Verification items for the finished model (mm, model axes). Face numbers are marked on the shaded views. A direction names the side the tool comes from. Give positions to 0.01 mm unless a question says otherwise; leave off trailing zeros. Order: outer loops, then holes, each group sorted by start corner. A loop starts at its lowest first (then second) coordinate and runs counter-clockwise, first axis right, second up. Notation, with made-up numbers: (-37.5, 46) -> (8.5, 46) arc R20 cw to (8.5, 64) -> close; hole circle Ø11 at (74.25, 50). An arc over 180 degrees is marked (long way). One line per question, with ' | ' between items. Start each with the question number.
Q1. Go/stop test with flat-tipped pins: pin 1 (1 mm diameter, centred on x = 40, z = -6.5, fed in from -Y); pin 2 (5 mm diameter, centred on x = 60, y = 23.5, fed in from +Z); pin 3 (13.5 mm diameter, centred on x = 62.5, z = -3.5, fed in from +Y). Record where each tip stops, or that it passes through.
Q2. Material ranges on probe 1 along Y at (x, z) = (-16.5, 2); probe 2 along Y at (x, z) = (7, -6.5); probe 3 along X at (y, z) = (2.5, -8), recorded low to high. Write a range as [from, to].
Q3. Access from +Z, -Z, +X, -X, +Y, -Y to the whole of each face (thin tool, end or side, straight path). Record for the marked faces 5, 6 and 7.
Q4. Mould release check, pull along Y, two halves, no side actions. Record for the marked faces 1, 2, 3 and 4: released by +Y, released by -Y, zero draft, split by the parting line, or undercut.
Q5. Section check B-B on y = -35. Record the cut outline in (x, z), plus the area to 3 significant figures.
Q6. Section check A-A on x = 7. Record the cut outline in (y, z), plus the area to 3 significant figures.
from build123d import *

# Parameters (mm, degrees)
SKETCH001_W          = 113
SKETCH001_H          = 85
PAD001_DEPTH         = 25
POCKET_DEPTH         = 36.5
SKETCH003_W          = 67.1
SKETCH003_H          = 19.5
POCKET001_DEPTH      = 61.5
POCKET002_DEPTH      = 17.5
SKETCH005_W          = 4
SKETCH005_H          = 8
SKETCH005_W_2        = 10
SKETCH005_H_2        = 10
POCKET003_DEPTH      = 42.501
POCKET003_DEPTH_BACK = 42.501
SKETCH006_W          = 3.6
SKETCH006_H          = 6
POCKET004_DEPTH      = 17
SKETCH007_W          = 250
SKETCH007_H          = 80
POCKET005_DEPTH      = 112.501
SKETCH008_R          = 30
POCKET006_DEPTH      = 32
POCKET007_DEPTH      = 18.5
POCKET008_DEPTH      = 25
SKETCH012_W          = 37.5
SKETCH012_H          = 25
POCKET009_DEPTH      = 20
SKETCH026_W          = 5
SKETCH026_H          = 10
PAD008_DEPTH         = 5
POCKET014_DEPTH      = 63.501
POCKET015_DEPTH      = 15
SKETCH029_W          = 1.43005
SKETCH029_H          = 20
PAD009_DEPTH         = 20
POCKET016_DEPTH      = 9
CHAMFER_SIZE         = 3
POCKET017_DEPTH      = 15
SKETCH032_W          = 21
SKETCH032_H          = 11.5
POCKET018_DEPTH      = 41


with BuildPart() as part:
    # Sketch001 → Pad001 (new body, symmetric)
    with BuildSketch(Plane.XY):
        with Locations((26.5, 0)):
            Rectangle(SKETCH001_W, SKETCH001_H)
    extrude(amount=PAD001_DEPTH, both=True)

    # Sketch002 (on DatumPlane) → Pocket (cut)
    with BuildSketch(Plane.XZ.offset(70)):
        with BuildLine():
            ThreePointArc((0, -20), (10.954451, -16.733201), (18.330303, -8))
            Line((18.330303, -8), (55.5, -8))
            Line((55.5, -8), (55.5, 20))
            Line((55.5, 20), (-30, 20))
            Line((-30, 20), (-30, -20))
            Line((-30, -20), (0, -20))
        make_face()
    pocket = extrude(amount=-POCKET_DEPTH, mode=Mode.SUBTRACT)

    # Mirrored: Pocket across XZ
    add(pocket.mirror(Plane.XZ), mode=Mode.SUBTRACT)

    # Sketch003 (on DatumPlane) → Pocket001 (cut)
    with BuildSketch(Plane.XY.offset(50)):
        with Locations((21.95, -29.65)):
            Rectangle(SKETCH003_W, SKETCH003_H)
        with Locations((21.95, 29.65)):
            Rectangle(SKETCH003_W, SKETCH003_H)
    extrude(amount=-POCKET001_DEPTH, mode=Mode.SUBTRACT)

    # Sketch004 (on DatumPlane) → Pocket002 (cut, symmetric)
    with BuildSketch(Plane.XZ):
        Polygon((-21, 4.923702), (-9.5, -11.5), (77, -11.5), (77, 8.5), (74, 11.5), (74, 38.5), (-21, 38.5), (-21, 13.5), (-19, 13.5), (-19, 12.5), (-21, 10.5), align=None)
    extrude(amount=POCKET002_DEPTH, both=True, mode=Mode.SUBTRACT)

    # Sketch005 (on DatumPlane) → Pocket003 (cut, two sides)
    with BuildSketch(Plane.XZ) as pocket003_sk:
        with Locations((31, 0)):
            Rectangle(SKETCH005_W, SKETCH005_H)
        with Locations((50.5, 0)):
            Rectangle(SKETCH005_W_2, SKETCH005_H_2)
        with BuildLine():
            ThreePointArc((3.272614, 2.3), (-4, 0), (3.272614, -2.3))
            Line((11.25, -2.3), (3.272614, -2.3))
            ThreePointArc((11.25, -2.3), (13.55, 0), (11.25, 2.3))
            Line((11.25, 2.3), (3.272614, 2.3))
        make_face()
    extrude(amount=-POCKET003_DEPTH, mode=Mode.SUBTRACT)
    extrude(pocket003_sk.sketch, amount=POCKET003_DEPTH_BACK, mode=Mode.SUBTRACT)

    # Sketch006 (on DatumPlane) → Pocket004 (cut)
    with BuildSketch(Plane.YZ):
        with Locations((-30, 0)):
            Rectangle(SKETCH006_W, SKETCH006_H)
        with Locations((30, 0)):
            Rectangle(SKETCH006_W, SKETCH006_H)
    extrude(amount=-POCKET004_DEPTH, mode=Mode.SUBTRACT)

    # Sketch007 (on DatumPlane) → Pocket005 (cut, through all)
    with BuildSketch(Plane.XZ.offset(70)):
        Rectangle(SKETCH007_W, SKETCH007_H)
        Polygon((-11.5, -13.5), (78, -13.5), (83, -8.5), (83, 13.5), (78.690599, 13.5), (78.690599, 14.5), (81, 18.5), (74, 18.5), (74, 13.5), (-3, 13.5), (-3, 17.5), (-7, 17.5), (-11, 13.5), (-23, 13.5), (-23, 2.923702), align=None, mode=Mode.SUBTRACT)
    extrude(amount=-POCKET005_DEPTH, mode=Mode.SUBTRACT)

    # Sketch008 (on DatumPlane) → Pocket006 (cut)
    with BuildSketch(Plane.XZ.offset(70)):
        with Locations((73, 7.4)):
            Circle(SKETCH008_R)
    pocket006 = extrude(amount=-POCKET006_DEPTH, mode=Mode.SUBTRACT)

    # Mirrored001: Pocket006 across XZ
    add(pocket006.mirror(Plane.XZ), mode=Mode.SUBTRACT)

    # Sketch009 (on DatumPlane) → Pocket007 (cut)
    with BuildSketch(Plane.XZ.offset(38)):
        Polygon((73, 10.9), (67.370835, 7.65), (67.370835, 1.15), (73, -2.1), (78.629165, 1.15), (78.629165, 7.65), align=None)
    pocket007 = extrude(amount=-POCKET007_DEPTH, mode=Mode.SUBTRACT)

    # Sketch010 (on DatumPlane) → Pocket008 (cut)
    with BuildSketch(Plane.YZ.offset(83)):
        Polygon((-27.1, 10.6), (-25.1, 8.6), (-23.1, 10.6), (-19.1, 10.6), (-21.986751, 15.6), (-28.213249, 15.6), (-31.1, 10.6), align=None)
    pocket008 = extrude(amount=-POCKET008_DEPTH, mode=Mode.SUBTRACT)

    # Sketch012 (on DatumPlane) → Pocket009 (cut)
    with BuildSketch(Plane.YZ.offset(83)):
        with Locations((-31.25, 26)):
            Rectangle(SKETCH012_W, SKETCH012_H)
        with Locations((31.25, 26)):
            Rectangle(SKETCH012_W, SKETCH012_H)
    extrude(amount=-POCKET009_DEPTH, mode=Mode.SUBTRACT)

    # Mirrored002: Pocket007 across XZ
    add(pocket007.mirror(Plane.XZ), mode=Mode.SUBTRACT)

    # Mirrored003: Pocket008 across XZ
    add(pocket008.mirror(Plane.XZ), mode=Mode.SUBTRACT)

    # Sketch026 (on DatumPlane) → Pad008 (join, symmetric)
    with BuildSketch(Plane.XZ):
        with Locations((11.5, -6.5)):
            Rectangle(SKETCH026_W, SKETCH026_H)
    extrude(amount=PAD008_DEPTH, both=True)

    # Sketch027 (on DatumPlane) → Pocket014 (cut, through all)
    with BuildSketch(Plane.XY.offset(50)):
        Polygon((24, 0), (25.443376, -2.5), (28.330127, -2.5), (43.669873, -2.5), (46.556624, -2.5), (48, 0), (46.556624, 2.5), (43.669873, 2.5), (28.330127, 2.5), (25.443376, 2.5), align=None)
    extrude(amount=-POCKET014_DEPTH, mode=Mode.SUBTRACT)

    # Sketch028 (on DatumPlane) → Pocket015 (cut)
    with BuildSketch(Plane.YZ.offset(83)):
        Polygon((-4.5, -1.65), (-3.200962, -3.9), (-0.602886, -3.9), (0.602886, -3.9), (3.200962, -3.9), (4.5, -1.65), (3.200962, 0.6), (0.602886, 0.6), (-0.602886, 0.6), (-3.200962, 0.6), align=None)
        Polygon((-7.5, 10), (-5.479274, 6.5), (-1.437822, 6.5), (1.437822, 6.5), (5.479274, 6.5), (7.5, 10), (5.479274, 13.5), (1.437822, 13.5), (-1.437822, 13.5), (-5.479274, 13.5), align=None)
    extrude(amount=-POCKET015_DEPTH, mode=Mode.SUBTRACT)

    # Sketch029 (on DatumPlane) → Pad009 (join)
    with BuildSketch(Plane(origin=(77, 0, 0), x_dir=(0, -1, 0), z_dir=(-1, 0, 0))):
        with Locations((-16.715025, -1.5)):
            Rectangle(SKETCH029_W, SKETCH029_H)
        with Locations((16.715025, -1.5)):
            Rectangle(SKETCH029_W, SKETCH029_H)
    extrude(amount=PAD009_DEPTH)

    # Sketch030 (on DatumPlane) → Pocket016 (cut, symmetric)
    with BuildSketch(Plane.XZ):
        Polygon((83, 3.486751), (78, 0.6), (78, -3.9), (83, -6.786751), align=None)
    extrude(amount=POCKET016_DEPTH, both=True, mode=Mode.SUBTRACT)

    # Chamfer
    chamfer_edges = [part.edges().sort_by_distance(p)[0] for p in [
        (78, -9, -1.65),
        (78, 9, -1.65),
    ]]
    chamfer(chamfer_edges, length=CHAMFER_SIZE)

    # Sketch031 (on DatumPlane) → Pocket017 (cut)
    with BuildSketch(Plane(origin=(-30, 0, 0), x_dir=(0, -1, 0), z_dir=(-1, 0, 0))):
        Polygon((-17.5, 13.5), (-13.5, 3), (-6, 13.5), align=None)
        Polygon((6, 13.5), (13.5, 3), (17.5, 13.5), align=None)
    extrude(amount=-POCKET017_DEPTH, mode=Mode.SUBTRACT)

    # Sketch032 (on DatumPlane) → Pocket018 (cut)
    with BuildSketch(Plane.XY.offset(50)):
        with Locations((-10.5, 11.75)):
            Rectangle(SKETCH032_W, SKETCH032_H)
        with Locations((-10.5, -11.75)):
            Rectangle(SKETCH032_W, SKETCH032_H)
    extrude(amount=-POCKET018_DEPTH, mode=Mode.SUBTRACT)


solid = part.part
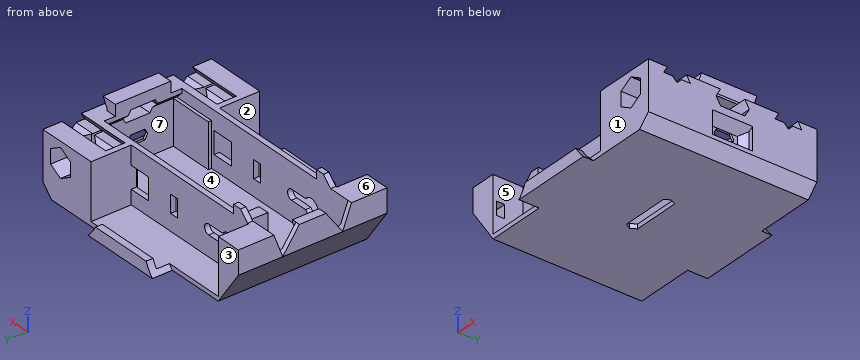
Filled in:
1) pin 1: y = -19.9 | pin 2: z = 13.5 | pin 3: y = 38
2) probe 1: [-33.5, -31.8], [-28.2, -17.5], [17.5, 28.2], [31.8, 33.5] | probe 2: [-19.9, -17.5], [17.5, 19.9] | probe 3: [-15.35, -11.95], [9, 14], [77, 83]
3) face 5: +Z, -Y | face 6: +Z, -X, +Y, -Y | face 7: none
4) face 1: released by -Y | face 2: zero draft | face 3: released by +Y | face 4: undercut
5) outline: (14.76, -13.5) -> (78, -13.5) -> (83, -8.5) -> (83, 13.5) -> (55.5, 13.5) -> (55.5, -11.5) -> (16.36, -11.5) arc R20 cw to start; hole (67.37, 1.15) -> (73, -2.1) -> (78.63, 1.15) -> (78.63, 7.65) -> (73, 10.9) -> (67.37, 7.65) -> close | area: 700 mm²
6) outline: (-33.5, -13.5) -> (33.5, -13.5) -> (33.5, -11.5) -> (19.9, -11.5) -> (19.9, -2.3) -> (17.5, -2.3) -> (17.5, -11.5) -> (-17.5, -11.5) -> (-17.5, -2.3) -> (-19.9, -2.3) -> (-19.9, -11.5) -> (-33.5, -11.5) -> close; (-19.9, 2.3) -> (-17.5, 2.3) -> (-17.5, 13.5) -> (-19.9, 13.5) -> close; (17.5, 2.3) -> (19.9, 2.3) -> (19.9, 13.5) -> (17.5, 13.5) -> close | area: 232 mm²
